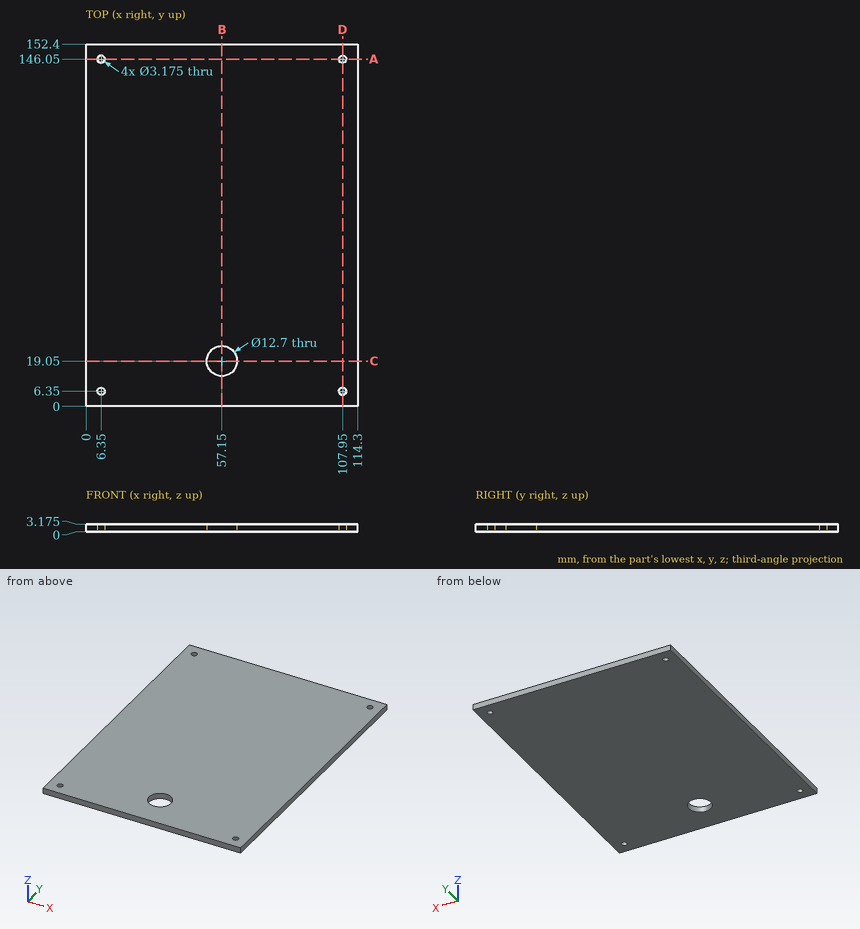
Can you work these out from the drawing? Everything is in mm from the part's minimum corner. Round coordinates to 2 decimals unless told otherwise and drop trailing zeros. Write each loop counter-clockwise with the first axis right and the second up, starting at its lowest first coordinate (ties: lowest second). Pieces come first, ordered by that corner, then holes. Notation, with made-up numbers: (72.25, -7) - (79.25, -7) arc R25 ccw to (79.25, 13) - close; hole circle Ø2 at (69.5, 22). An arc over 180 degrees is marked (long way). Put each result on its own line as item: value. Start each with the question number.
(1) Will this pin go through, and if not, where does the flat tip stop? pin 1 (1.9 mm diameter, centred on x = 107.95, y = 6.35, fed in from +Z).
(2) I want a section at C-C, the plane y = 19.05. Please give me the cut outline in (x, z) (3 decimals), plus the area to 3 significant figures.
(3) I want a section at B-B, the plane x = 57.15. Please give me the cut outline in (y, z) (3 decimals).
(4) I want a section at A-A, the plane y = 146.05. Please give me the cut outline in (x, z) (1 decimal).
(5) I need wall thicknesses on probe 1 along X at (y, z) = (146.05, 1.4); probe 2 along Y at (x, z) = (107.95, 1.9); probe 3 along X at (y, z) = (19.05, 0.7). Which ranges of each line are inside material? Lowest first, please.
(6) I want a section at D-D, the plane x = 107.95. Please give me the cut outline in (y, z) (1 decimal), plus the area to 3 significant figures.
Here are the results:
1. pin 1: passes through
2. outline: (0, 0) - (50.8, 0) - (50.8, 3.175) - (0, 3.175) - close; (63.5, 0) - (114.3, 0) - (114.3, 3.175) - (63.5, 3.175) - close
2. area: 323 mm^2
3. outline: (0, 0) - (12.7, 0) - (12.7, 3.175) - (0, 3.175) - close; (25.4, 0) - (152.4, 0) - (152.4, 3.175) - (25.4, 3.175) - close
4. outline: (0, 0) - (4.8, 0) - (4.8, 3.2) - (0, 3.2) - close; (7.9, 0) - (106.4, 0) - (106.4, 3.2) - (7.9, 3.2) - close; (109.5, 0) - (114.3, 0) - (114.3, 3.2) - (109.5, 3.2) - close
5. probe 1: x = 0 to 4.76, 7.94 to 106.36, 109.54 to 114.3
5. probe 2: y = 0 to 4.76, 7.94 to 144.46, 147.64 to 152.4
5. probe 3: x = 0 to 50.8, 63.5 to 114.3
6. outline: (0, 0) - (4.8, 0) - (4.8, 3.2) - (0, 3.2) - close; (7.9, 0) - (144.5, 0) - (144.5, 3.2) - (7.9, 3.2) - close; (147.6, 0) - (152.4, 0) - (152.4, 3.2) - (147.6, 3.2) - close
6. area: 464 mm^2
